For this review, take the finished solid that the model builds, in its own axes (mm). Face numbers are marked on the shaded views. A direction names the side the tool comes from. Give positions to 0.01 mm unless a question says otherwise; leave off trailing zeros. Loops run counter-clockwise (first coordinate to the right, second up) from the corner with the lowest first, then second, coordinate; pieces in that order, holes last. Notation, with made-up numbers: (69.5, 3) -> (92.5, 3) arc R27 cw to (92.5, 29) -> close; hole circle Ø4 at (-27.75, 74). An arc over 180 degrees is marked (long way). Write each question's results on one line, items separated by ' | '. Start each with the question number.
```python
from build123d import *

# Parameters (mm, degrees)
F0_W      = 25.4
F0_H      = 50.8
F1_DEPTH  = 25.4
F5_DEPTH  = 25.4
F6_DEPTH  = 25.4
F4_W      = 3.81
F4_H      = 3.81
F7_DEPTH  = 50.8
F9_DEPTH  = 25.4
F10_W     = 4.259707
F10_H     = 4.259707
F11_DEPTH = 25.4
F12_DEPTH = 25.4
F13_DEPTH = 25.4


with BuildPart() as f1:
    # F0 (on Right) → F1 (new body)
    with BuildSketch(Plane.YZ):
        Rectangle(F0_W, F0_H)
    extrude(amount=F1_DEPTH)

    # F2 (on face) → F5 (cut)
    with BuildSketch(Plane(origin=(0, 0, 0), x_dir=(0, -1, 0), z_dir=(-1, 0, 0))):
        Polygon((8.4402905029, 0), (0, 16.8805810057), (-8.4402905029, 0), (0, -16.8805810057), align=None)
    extrude(amount=-F5_DEPTH, mode=Mode.SUBTRACT)

    # F3 (on face) → F6 (cut)
    with BuildSketch(Plane(origin=(0, 12.7, 0), x_dir=(-1, 0, 0), z_dir=(0, 1, 0))):
        Polygon((-12.7, 16.8805810057), (-21.1402905029, 0), (-12.7, -16.8805810057), (-4.2597094971, 0), align=None)
    extrude(amount=-F6_DEPTH, mode=Mode.SUBTRACT)

    # F4 (on face) → F7 (join)
    with BuildSketch(Plane(origin=(0, 0, -25.4), x_dir=(1, 0, 0), z_dir=(0, 0, -1))):
        with Locations((12.7, 0)):
            Rectangle(F4_W, F4_H)
    extrude(amount=-F7_DEPTH)

    # F8 (on face) → F9 (join)
    with BuildSketch(Plane.YZ.offset(25.4)):
        Polygon((-12.7, 2.1298535), (-12.7, -2.1298535), (-8.4402905029, -2.1298535), (-8.4402905029, 0), (-8.4402905029, 2.1298535), align=None)
        Polygon((8.4402905029, -2.1298535), (12.7, -2.1298535), (12.7, 2.1298535), (8.4402905029, 2.1298535), (8.4402905029, 0), align=None)
    extrude(amount=-F9_DEPTH)

    # F10 (on face) → F11 (join)
    with BuildSketch(Plane.XZ.offset(12.7)):
        with Locations((2.1298535, 0)):
            Rectangle(F10_W, F10_H)
        with Locations((23.2701465, 0)):
            Rectangle(F10_W, F10_H)
    extrude(amount=-F11_DEPTH)

    # F3 (on face) → F12 (cut)
    with BuildSketch(Plane(origin=(0, 12.7, 0), x_dir=(-1, 0, 0), z_dir=(0, 1, 0))):
        Polygon((0, 25.4), (-12.7, 25.4), (0, 0), align=None)
        Polygon((-25.4, 0), (-12.7, 25.4), (-25.4, 25.4), align=None)
        Polygon((-12.7, -25.4), (-25.4, 0), (-25.4, -25.4), align=None)
        Polygon((0, -25.4), (0, 0), (-12.7, -25.4), align=None)
    extrude(amount=-F12_DEPTH, mode=Mode.SUBTRACT)

    # F2 (on face) → F13 (cut)
    with BuildSketch(Plane(origin=(0, 0, 0), x_dir=(0, -1, 0), z_dir=(-1, 0, 0))):
        Polygon((-12.7, 0), (0, 25.4), (-12.7, 25.4), align=None)
        Polygon((12.7, 25.4), (0, 25.4), (12.7, 0), align=None)
        Polygon((12.7, -25.4), (12.7, 0), (0, -25.4), align=None)
        Polygon((0, -25.4), (-12.7, 0), (-12.7, -25.4), align=None)
    extrude(amount=-F13_DEPTH, mode=Mode.SUBTRACT)


solid = f1.part
```
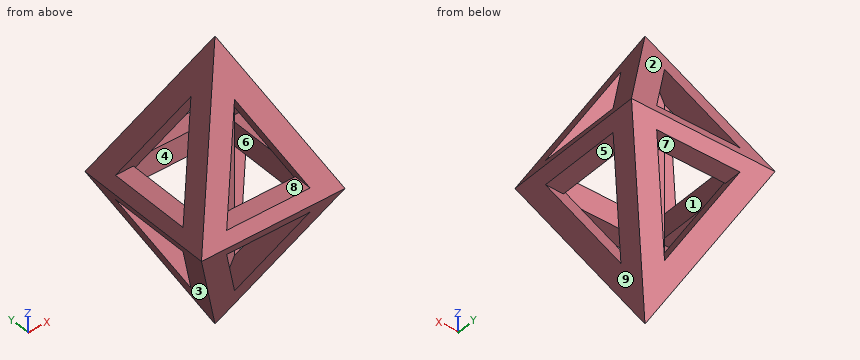
1. Machinability: for the marked faces 5, 6, 7, 8 and 9, which of the approach directions +Z, -Z, +X, -X, +Y, -Y give a long, thin tool a straight path to every point of the face, cutting with its end or side? Answer none if there is none.
2. For pin 1 Ø1 at (x, y) = (3, 0) entering from -Z; pin 2 Ø12 at (y, z) = (-5.5, -18.5) entering from +X; pin 3 Ø4 at (x, z) = (13.5, -17.5) entering from -Y, all flat-tipped, find the tip position at first contact; note any pin that passes through.
3. We need section C-C (x = 12). Write out the cut boundary in (y, z) (3 decimals), plus the area to 3 significant figures.
4. We need section A-A (x = 18.25). Write out the cut boundary in (y, z).
5. We need section D-D (y = -6). Write out the cut boundary in (x, z).
6. We need section B-B (z = 5). Write out the cut boundary in (x, y) (3 decimals), plus the area to 3 significant figures.
7. Wall thickness on L1, parallel to Y at x = 11, z = 1 (3 decimals); L2, parallel to X at y = 3.75, z = -1; L3, parallel to Z at x = 11.5, y = 11.25: over which ranges is each line inside the solid? List them lowest first.
8. Draft analysis for pull direction X (two halves, no side actions). For the marked faces 1, 2, 3 and 4, state which applies: released by +X, released by -X, zero draft, split by the parting line, or undercut.
Response:
1) face 5: +X | face 6: none | face 7: +Y | face 8: -Y | face 9: -Z, +X, +Y, -Y
2) pin 1: stops at z = -2.13 | pin 2: stops at x = 19.15 | pin 3: stops at y = -4.95
3) outline: (-12.7, 0) -> (-11.635, -2.13) -> (-8.44, -2.13) -> (-8.44, 2.13) -> (-11.635, 2.13) -> close; (-4.96, -15.481) -> (-0.7, -24) -> (0.7, -24) -> (4.96, -15.481) -> (1.905, -15.481) -> (1.905, 15.481) -> (4.96, 15.481) -> (0.7, 24) -> (-0.7, 24) -> (-4.96, 15.481) -> (-1.905, 15.481) -> (-1.905, -15.481) -> close; (8.44, -2.13) -> (11.635, -2.13) -> (12.7, 0) -> (11.635, 2.13) -> (8.44, 2.13) -> close | area: 246 mm2
4) outline: (-12.7, 0) -> (-11.64, -2.13) -> (-8.44, -2.13) -> (-8.44, 2.13) -> (-11.64, 2.13) -> close; (-9.81, -5.78) -> (-5.55, -14.3) -> (-1.29, -14.3) -> (-5.55, -5.78) -> close; (-9.81, 5.78) -> (-5.55, 5.78) -> (-1.29, 14.3) -> (-5.55, 14.3) -> close; (1.29, -14.3) -> (5.55, -14.3) -> (9.81, -5.78) -> (5.55, -5.78) -> close; (1.29, 14.3) -> (5.55, 5.78) -> (9.81, 5.78) -> (5.55, 14.3) -> close; (8.44, -2.13) -> (11.64, -2.13) -> (12.7, 0) -> (11.64, 2.13) -> (8.44, 2.13) -> close
5) outline: (0, 0) -> (1.06, -2.13) -> (4.26, -2.13) -> (4.26, 2.13) -> (1.06, 2.13) -> close; (2.44, -4.88) -> (6.7, -13.4) -> (10.96, -13.4) -> (6.7, -4.88) -> close; (2.44, 4.88) -> (6.7, 4.88) -> (10.96, 13.4) -> (6.7, 13.4) -> close; (14.44, -13.4) -> (18.7, -13.4) -> (22.96, -4.88) -> (18.7, -4.88) -> close; (14.44, 13.4) -> (18.7, 4.88) -> (22.96, 4.88) -> (18.7, 13.4) -> close; (21.14, -2.13) -> (24.34, -2.13) -> (25.4, 0) -> (24.34, 2.13) -> (21.14, 2.13) -> close
6) outline: (2.5, -10.2) -> (6.76, -10.2) -> (6.76, -5.94) -> (2.5, -5.94) -> close; (2.5, 5.94) -> (6.76, 5.94) -> (6.76, 10.2) -> (2.5, 10.2) -> close; (10.795, -1.905) -> (14.605, -1.905) -> (14.605, 1.905) -> (10.795, 1.905) -> close; (18.64, -10.2) -> (22.9, -10.2) -> (22.9, -5.94) -> (18.64, -5.94) -> close; (18.64, 5.94) -> (22.9, 5.94) -> (22.9, 10.2) -> (18.64, 10.2) -> close | area: 87.1 mm2
7) L1: y = -12.2 to -8.44, -1.905 to 1.905, 8.44 to 12.2 | L2: x = 0.5 to 4.26, 21.14 to 24.9 | L3: z = -2.13 to 2.13
8) face 1: undercut | face 2: zero draft | face 3: released by -X | face 4: undercut
